For this review, use the dimensioned drawing (mm, ordinates from the lowest corner) and the shaded views. Give positions to 0.01 mm unless a question says otherwise; leave off trailing zeros. Write each loop counter-clockwise with the first axis right and the second up, starting at its lowest first coordinate (ties: lowest second). Pieces come first, ordered by that corner, then holes. Notation, with made-up numbers: M -22.5,83.5 L -10.5,83.5 A29 ccw -10.5,112.5 Z; hole C 58,29 d11. An arc over 180 degrees is marked long. Answer in a Markdown table with one row per item.
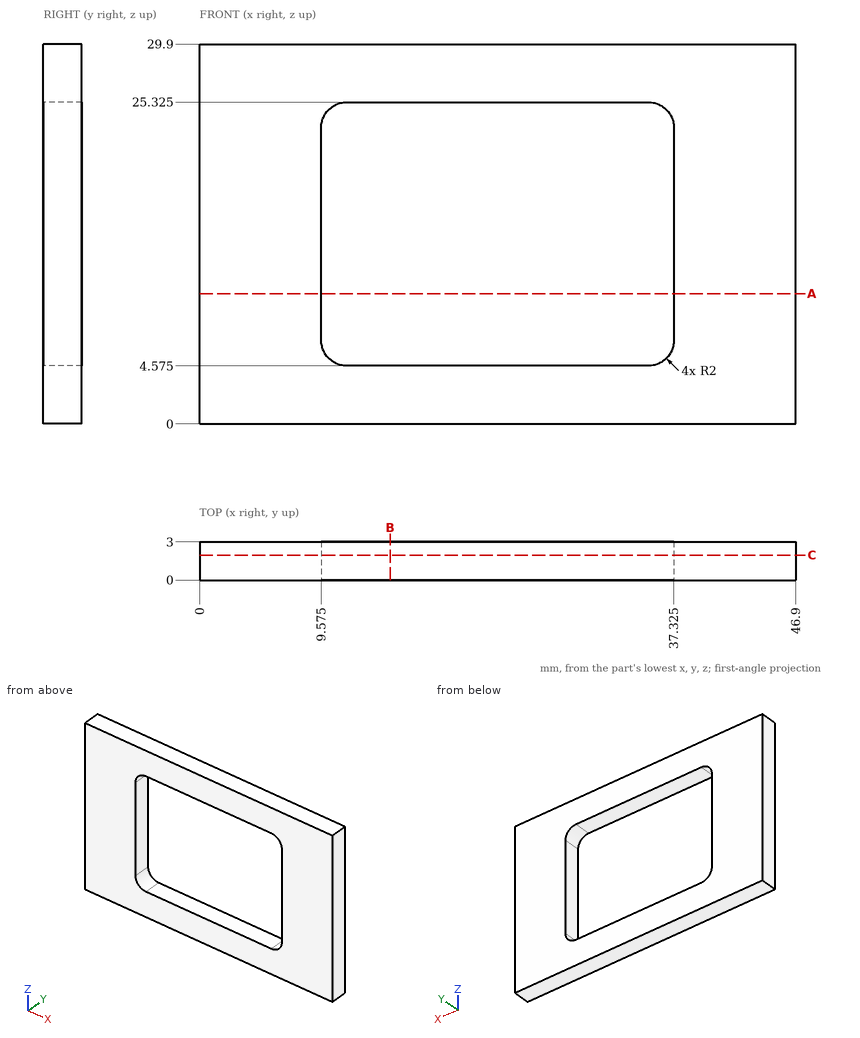
1) To check wall thickness, follow probe 1 along X at (y, z) = (2.1, 18) (3 decimals); probe 2 along Z at (x, y) = (26, 1.05) (3 decimals). State the ranges of each line that lie inside material, in increasing order. Write a range as [from, to].
Geometry says:
| item | result |
|---|---|
| probe 1 | [0, 9.575], [37.325, 46.9] |
| probe 2 | [0, 4.575], [25.325, 29.9] |
2) Insertion check: P1, Ø0.9, axis at x = 18.5, y = 1.5, coming from the -Z side. The pin has a flat end and moves straight along its axis. Give the tip position at first contact, or say it passes through.
Geometry says:
| item | result |
|---|---|
| P1 | z = 0 |
3) Add section B-B (x = 15). Write out the cut boundary in (y, z) (3 decimals).
Geometry says:
| item | result |
|---|---|
| outline | M 0,0 L 3,0 L 3,4.575 L 0,4.575 Z; M 0,25.325 L 3,25.325 L 3,29.9 L 0,29.9 Z |
4) Add section C-C (y = 1.95). Write out the cut boundary in (x, z) (3 decimals), and give its area (3 significant figures).
Geometry says:
| item | result |
|---|---|
| outline | M 0,0 L 46.9,0 L 46.9,29.9 L 0,29.9 Z; hole M 9.575,6.575 A2 ccw 11.575,4.575 L 35.325,4.575 A2 ccw 37.325,6.575 L 37.325,23.325 A2 ccw 35.325,25.325 L 11.575,25.325 A2 ccw 9.575,23.325 Z |
| area | 830 mm^2 |
5) Add section A-A (z = 10.25). Write out the cut boundary in (x, y) (3 decimals).
Geometry says:
| item | result |
|---|---|
| outline | M 0,0 L 9.575,0 L 9.575,3 L 0,3 Z; M 37.325,0 L 46.9,0 L 46.9,3 L 37.325,3 Z |
